For this review, take the finished solid that the model builds, in its own axes (mm). A direction names the side the tool comes from. Round coordinates to 2 decimals unless told otherwise and drop trailing zeros. Write each loop counter-clockwise with the first axis right and the second up, starting at its lowest first coordinate (ties: lowest second). Pieces come first, ordered by that corner, then holes. Notation, with made-up numbers: (1.25, 12.25) - (39.25, 12.25) arc R19 ccw to (39.25, 19.25) - close; hole circle Ø7 at (69.25, 47.5). An arc over 180 degrees is marked (long way). One line per item, written item: value. Start each with the question number.
Q1. For probe 1 along Y at (x, z) = (1.35, 3.5); probe 2 along Z at (x, y) = (1.4, 5); probe 3 along Y at (x, z) = (1.9, -14), list the stretches that pass through material, from the lowest coordinate up.
Q2. Tool access review of faces 1 (the face through (1.676, -8.839, 2.106)), 2 (the face through (1.324, 2.106, -8.839)), 3 (the face through (2, -7, 1.5)): name each direction out of +Z, -Z, +X, -X, +Y, -Y from which nothing blocks a thin tool from reaching the whole face with its end or side.
Q3. Add section C-C on y = -7.5. Write out the cut boundary in (x, z), and give its area (3 significant figures).
Q4. Add section A-A on x = 1.5. Write out the cut boundary in (y, z).
Q5. Add section D-D on z = 0.5. Write out the cut boundary in (x, y), and give its area (3 significant figures).
Q6. Clearance check with flat-ended pins moving along their axes: pin 1 Ø1.5 at (x, z) = (0.5, 11.5) entering from +Y; pin 2 Ø6 at (y, z) = (14.5, -10) entering from -X; pin 3 Ø1.5 at (x, z) = (1, -6) entering from -Y; pin 4 Ø1.2 at (x, y) = (1.5, -7.5) entering from -Z. State where each tip first meets the part, or that it passes through.
Q7. Add section B-B on z = -7.5. Write out the cut boundary in (x, y).
Q8. Mouldability with a two-part tool opening along Z and no side actions: class faces 4 (the face through (2, 3, -16.796)), 5 (the face through (2.8, 2.5, -8.3)), 6 (the face through (1, 1.5, -7)), 7 (the face through (1.479, 1.748, 1.787)) as +Z half, -Z half, draft (parallel to the pull), parting line (faces both ways), or undercut.
Autodesk Inventor part; units mm, degrees
ref_plane "YZ Plane" through (0, 0, 0) normal (1, 0, 0) x (0, 1, 0)
ref_plane "XZ Plane" through (0, 0, 0) normal (0, 1, 0) x (-1, 0, 0)
ref_plane "XY Plane" through (0, 0, 0) normal (0, 0, 1) x (1, 0, 0)
sketch "Boceto1" plane through (0, 0, 0) normal (1, 0, 0) x (0, 1, 0)
  circle A0 centre (0, 0) radius 2.5
  line L0 (2.5, 0) -> (2.5, 10.6639)
  line L1 (2.5, 2.5) -> (-7.5, 2.5)
  line L2 (-7.5, 2.5) -> (-9.5, 2.5)
  line L3 (-9.5, 2.5) -> (-9.5, 4.5)
  line L4 (-9.5, 4.5) -> (2.5, 4.5)
  line L5 (0, 0) -> (-4.5773, -4.5773)
  line L6 (0, 0) -> (6.4732, 0) construction
  circle A1 centre (0, 0) radius 2.5
  line L7 (0, 2.5) -> (10.6639, 2.5)
  line L8 (2.5, 2.5) -> (2.5, -7.5)
  line L9 (2.5, -7.5) -> (2.5, -9.5)
  line L10 (2.5, -9.5) -> (4.5, -9.5)
  line L11 (4.5, -9.5) -> (4.5, 2.5)
  line L12 (2.5, 4.5) -> (4.5, 4.5)
  line L13 (4.5, 4.5) -> (4.5, 2.5)
  point P0 (0, 2.5)
  dimension "d0" = 5
  dimension "d1" = 10
  dimension "d2" = 2
  dimension "d3" = 2
  dimension "d4" = 135
extrude "Extrusión1" add sketch "Boceto1" along normal blind 3 contours A0 L1 L0 | L0 L7 L11 L10 L9 L8 | L1 L2 L3 L4 L0 | L0 L12 L13 L7
sketch "Boceto2" plane through (3, 0, 0) normal (1, 0, 0) x (0, 0, -1)
  line L0 (16.7965, 4.5) -> (-17.9745, 33.0686)
  line L1 (-4.5, 4.5) -> (-4.5, -9.5)
  line L2 (-17.9745, 33.0686) -> (-4.5, -9.5)
  line L3 (-2.5, -9.5) -> (-2.5, 0)
  arc A0 (0, 2.5) -> (-2.5, 0) centre (0, 0) ccw
  line L4 (0, 2.5) -> (9.5, 2.5)
  line L5 (9.5, 2.5) -> (9.5, 4.5)
  line L6 (9.5, 4.5) -> (-4.5, 4.5)
  line L7 (-4.5, 4.5) -> (-4.5, -9.5)
  line L8 (-4.5, -9.5) -> (-2.5, -9.5)
  line L9 (9.5, 2.5) -> (9.5, 4.5)
  line L10 (9.5, 4.5) -> (16.7965, 4.5)
  line L11 (16.7965, 2.5) -> (9.5, 2.5)
  line L12 (9.5, 2.5) -> (16.7965, 2.5)
  line L13 (16.7965, 4.5) -> (16.7965, 2.5)
extrude "Extrusión2" add sketch "Boceto2" against normal blind 3 contours L10 L6 L1 L2 L0 | L13 L11 L5 L10
sketch "Boceto3" plane through (0, 2.5, -9.5) normal (0, -1, 0) x (1, 0, 0)
  line L0 (0, 0) -> (3, 0)
  line L1 (1.5, 0) -> (1.5, 2)
  circle A0 centre (1.5, 2) radius 1.35
  point P0 (0, 9.5)
  dimension "d9" = 2
  dimension "d10" = 2.7
extrude "Extrusión3" add sketch "Boceto3" along normal blind 1
fillet "Empalme1" radius 0.2 1 edges at (0.15, 1.5, -7.5)
sketch "Boceto4" plane through (0, -9.5, 2.5) normal (0, 0, -1) x (-1, 0, 0)
  line L0 (0, 0) -> (-3, 0)
  line L1 (-1.5, 0) -> (-1.5, 2)
  circle A0 centre (-1.5, 2) radius 1.35
  point P0 (0, 9.5)
  dimension "d14" = 2
  dimension "d15" = 2.7
extrude "Extrusión4" add sketch "Boceto4" along normal blind 1
fillet "Empalme2" radius 0.2 1 edges at (2.85, -7.5, 1.5)
fillet "Empalme3" radius 1 3 edges at (1.5, 4.5, -16.7965) (1.5, -9.5, 4.5) (1.5, 33.0686, 17.9745)
properties part number "gato"
Result set:
1. probe 1: y = -9.5 to 21.18
1. probe 2: z = -16.19 to 9.09
1. probe 3: y = 2.5 to 6.8
2. face 1: -Z
2. face 2: -Y
2. face 3: -Z, +X, -X, -Y
3. outline: (0, 2.5) - (0.15, 2.5) - (0.15, 1.7) arc R0.2 ccw to (0.35, 1.5) - (2.65, 1.5) arc R0.2 ccw to (2.85, 1.7) - (2.85, 2.5) - (3, 2.5) - (3, 5.13) - (0, 5.13) - close
3. area: 10.6 mm^2
4. outline: (-9.5, 2.5) - (-8.85, 2.5) - (-8.85, 1.7) arc R0.2 ccw to (-8.65, 1.5) - (-6.35, 1.5) arc R0.2 ccw to (-6.15, 1.7) - (-6.15, 2.5) - (0, 2.5) arc R2.5 cw to (2.5, 0) - (2.5, -6.15) - (1.7, -6.15) arc R0.2 ccw to (1.5, -6.35) - (1.5, -8.65) arc R0.2 ccw to (1.7, -8.85) - (2.5, -8.85) - (2.5, -16.8) - (4.03, -16.8) arc R1 ccw to (4.8, -16.43) - (30.93, 15.37) arc R1 ccw to (29.85, 16.96) - (-8.8, 4.72) arc R1 ccw to (-9.5, 3.77) - close
5. outline: (0, 2.45) - (3, 2.45) - (3, 18.71) - (0, 18.71) - close
5. area: 48.8 mm^2
6. pin 1: stops at y = 28.37
6. pin 2: passes through
6. pin 3: stops at y = 1.5
6. pin 4: stops at z = 1.5
7. outline: (0, 2.5) - (0.15, 2.5) - (0.15, 1.7) arc R0.2 ccw to (0.35, 1.5) - (2.65, 1.5) arc R0.2 ccw to (2.85, 1.7) - (2.85, 2.5) - (3, 2.5) - (3, 12.14) - (0, 12.14) - close
8. face 4: -Z half
8. face 5: undercut
8. face 6: draft
8. face 7: undercut
